For this review, take the finished solid that the model builds, in its own axes (mm). A direction names the side the tool comes from. Round coordinates to 2 decimals unless told otherwise and drop trailing zeros. Loops run counter-clockwise (first coordinate to the right, second up) from the corner with the lowest first, then second, coordinate; pieces in that order, holes last. Notation, with made-up numbers: M 48.25,76.25 L 81.25,76.25 A7 cw 81.25,87.25 Z; hole C 10,85 d7. An arc over 180 degrees is marked long. Write item = value, one per line. Start each with the question number.
```python
from build123d import *

# Parameters (mm, degrees)
BOSS_EXTRUDE1_DEPTH      = 8
BOSS_EXTRUDE1_DEPTH_BACK = 75
SKETCH3_W                = 2.5
SKETCH3_H                = 24
CUT_EXTRUDE1_DEPTH       = 10
BOSS_EXTRUDE6_DEPTH      = 90
BOSS_EXTRUDE6_DEPTH_BACK = 83
BOSS_EXTRUDE7_DEPTH      = 90
SKETCH8_W                = 7
SKETCH8_H                = 16.2
CUT_EXTRUDE2_DEPTH       = 15
SKETCH9_W                = 2
SKETCH9_H                = 12.2
CUT_EXTRUDE3_DEPTH       = 10
CUT_EXTRUDE4_DEPTH       = 90
CUT_EXTRUDE5_DEPTH       = 75
CUT_EXTRUDE6_DEPTH       = 90
CUT_EXTRUDE6_DEPTH_BACK  = 83
SKETCH13_R               = 1.75
SKETCH14_R               = 2
CUT_EXTRUDE7_DEPTH       = 83
SKETCH16_R               = 1.75
CUT_EXTRUDE8_DEPTH       = 3
CUT_EXTRUDE9_DEPTH       = 170
SKETCH18_R               = 2
CUT_EXTRUDE10_DEPTH      = 15
SKETCH19_W               = 8
SKETCH19_H               = 3
CUT_EXTRUDE11_DEPTH      = 3
CUT_EXTRUDE12_DEPTH      = 7
SKETCH21_W               = 7
SKETCH21_H               = 4.5
CUT_EXTRUDE13_DEPTH      = 17
SKETCH22_W               = 40
SKETCH22_H               = 42
CUT_EXTRUDE14_DEPTH      = 42
FILLET1_R                = 5


with BuildPart() as part:
    # Sketch2 → Boss-Extrude1 (new, two sides: drawn at the far end of the back side and taken through both)
    with BuildSketch(Plane(origin=(0, 0, 0), x_dir=(0, 0, -1), z_dir=(1, 0, 0)).offset(-BOSS_EXTRUDE1_DEPTH_BACK)):
        Polygon((-21, 0), (-21, 15), (-4, 15), (-4, 7), (0, 7), (4, 7), (4, 15), (21, 15), (21, 0), (0, 0), align=None)
    extrude(amount=BOSS_EXTRUDE1_DEPTH + BOSS_EXTRUDE1_DEPTH_BACK)

    # Sketch3 → Cut-Extrude1 (cut)
    with BuildSketch(Plane(origin=(0, 15, 0), x_dir=(-1, 0, 0), z_dir=(0, 1, 0))):
        with Locations((-3.75, 0)):
            Rectangle(SKETCH3_W, SKETCH3_H)
    extrude(amount=-CUT_EXTRUDE1_DEPTH, mode=Mode.SUBTRACT)

    # Sketch6 → Boss-Extrude6 (add, two sides: drawn at the far end of the back side and taken through both)
    with BuildSketch(Plane(origin=(8, 0, 0), x_dir=(0, 0, -1), z_dir=(1, 0, 0)).offset(-BOSS_EXTRUDE6_DEPTH_BACK)):
        Polygon((-12, 15), (-12, 0), (12, 0), (12, 15), (21, 15), (21, -27), (-21, -27), (-21, 15), align=None)
    extrude(amount=BOSS_EXTRUDE6_DEPTH + BOSS_EXTRUDE6_DEPTH_BACK)

    # Sketch7 → Boss-Extrude7 (add)
    with BuildSketch(Plane(origin=(8, 0, 0), x_dir=(0, 0, -1), z_dir=(1, 0, 0))):
        Polygon((2.25, 15), (2.25, 8.75), (-2.25, 8.75), (-2.25, 15), (-8.1, 15), (-8.1, 11), (-8.1, 0), (8.1, 0), (8.1, 11), (8.1, 15), align=None)
    extrude(amount=BOSS_EXTRUDE7_DEPTH)

    # Sketch8 → Cut-Extrude2 (cut)
    with BuildSketch(Plane(origin=(0, 15, 0), x_dir=(-1, 0, 0), z_dir=(0, 1, 0))):
        with Locations((-11.5, 0)):
            Rectangle(SKETCH8_W, SKETCH8_H)
    extrude(amount=-CUT_EXTRUDE2_DEPTH, mode=Mode.SUBTRACT)

    # Sketch9 → Cut-Extrude3 (cut)
    with BuildSketch(Plane(origin=(0, 15, 0), x_dir=(-1, 0, 0), z_dir=(0, 1, 0))):
        with Locations((-18, 0)):
            Rectangle(SKETCH9_W, SKETCH9_H)
    extrude(amount=-CUT_EXTRUDE3_DEPTH, mode=Mode.SUBTRACT)

    # Sketch11 → Cut-Extrude4 (cut)
    with BuildSketch(Plane(origin=(98, 0, 0), x_dir=(0, 0, -1), z_dir=(1, 0, 0))):
        with BuildLine():
            Line((4.5, 0), (8.1, 0))
            Line((8.1, 0), (8.1, 0.5))
            Line((8.1, 0.5), (4, 0.5))
            Line((4, 0.5), (4, 0))
            ThreePointArc((4, 0), (0, -4), (-4, 0))
            Line((-4, 0), (-4, 0.5))
            Line((-4, 0.5), (-8.1, 0.5))
            Line((-8.1, 0.5), (-8.1, 0))
            Line((-8.1, 0), (-4.5, 0))
            ThreePointArc((-4.5, 0), (0, -4.5), (4.5, 0))
        make_face()
    extrude(amount=-CUT_EXTRUDE4_DEPTH, mode=Mode.SUBTRACT)

    # Sketch12 → Cut-Extrude5 (cut)
    with BuildSketch(Plane(origin=(98, 0, 0), x_dir=(0, 0, -1), z_dir=(1, 0, 0))):
        with BuildLine():
            Line((-2.25, 15), (-8.1, 15))
            Line((-8.1, 15), (-8.1, 0.5))
            Line((-8.1, 0.5), (-4, 0.5))
            Line((-4, 0.5), (-4, 0))
            ThreePointArc((-4, 0), (0, -4), (4, 0))
            Line((4, 0), (4, 0.5))
            Line((4, 0.5), (8.1, 0.5))
            Line((8.1, 0.5), (8.1, 15))
            Line((8.1, 15), (2.25, 15))
            Line((2.25, 15), (2.25, 8.75))
            Line((2.25, 8.75), (-2.25, 8.75))
            Line((-2.25, 8.75), (-2.25, 15))
        make_face()
    extrude(amount=-CUT_EXTRUDE5_DEPTH, mode=Mode.SUBTRACT)

    # Sketch13 → Cut-Extrude6 (cut, two sides: drawn at the far end of the back side and taken through both)
    with BuildSketch(Plane(origin=(8, 0, 0), x_dir=(0, 0, -1), z_dir=(1, 0, 0)).offset(-CUT_EXTRUDE6_DEPTH_BACK)):
        Circle(SKETCH13_R)
    extrude(amount=CUT_EXTRUDE6_DEPTH + CUT_EXTRUDE6_DEPTH_BACK, mode=Mode.SUBTRACT)

    # Sketch14 → Cut-Extrude7 (cut)
    with BuildSketch(Plane(origin=(8, 0, 0), x_dir=(0, 0, -1), z_dir=(1, 0, 0))):
        Circle(SKETCH14_R)
    extrude(amount=-CUT_EXTRUDE7_DEPTH, mode=Mode.SUBTRACT)

    # Sketch16 → Cut-Extrude8 (cut)
    with BuildSketch(Plane(origin=(98, 0, 0), x_dir=(0, 0, -1), z_dir=(1, 0, 0))):
        with Locations((17.5, -8)):
            Circle(SKETCH16_R)
        with Locations((-17.5, -8)):
            Circle(SKETCH16_R)
    extrude(amount=-CUT_EXTRUDE8_DEPTH, mode=Mode.SUBTRACT)

    # Sketch17 → Cut-Extrude9 (cut)
    with BuildSketch(Plane(origin=(95, 0, 0), x_dir=(0, 0, -1), z_dir=(1, 0, 0))):
        Polygon((18, -6), (18, -27), (-18, -27), (-18, -6), (-4.5, -6), (-4.5, -9), (4.5, -9), (4.5, -6), align=None)
    extrude(amount=-CUT_EXTRUDE9_DEPTH, mode=Mode.SUBTRACT)

    # Sketch18 → Cut-Extrude10 (cut)
    with BuildSketch(Plane(origin=(95, 0, 0), x_dir=(0, 0, -1), z_dir=(1, 0, 0))):
        with Locations((-17.5, -8)):
            Circle(SKETCH18_R)
        with Locations((17.5, -8)):
            Circle(SKETCH18_R)
    extrude(amount=-CUT_EXTRUDE10_DEPTH, mode=Mode.SUBTRACT)

    # Sketch19 → Cut-Extrude11 (cut)
    with BuildSketch(Plane(origin=(95, 0, 0), x_dir=(0, 0, -1), z_dir=(1, 0, 0))):
        with Locations((0, -25.5)):
            Rectangle(SKETCH19_W, SKETCH19_H)
    extrude(amount=CUT_EXTRUDE11_DEPTH, mode=Mode.SUBTRACT)

    # Sketch20 → Cut-Extrude12 (cut)
    with BuildSketch(Plane(origin=(8, 0, 0), x_dir=(0, 0, -1), z_dir=(1, 0, 0))):
        with BuildLine():
            Line((-3.878333303, -1), (3.878323052, -1.000039756))
            ThreePointArc((3.878323052, -1.000039756), (-2.0528e-05, -4.005180297), (-3.878333303, -1))
        make_face()
    extrude(amount=CUT_EXTRUDE12_DEPTH, mode=Mode.SUBTRACT)

    # Sketch21 → Cut-Extrude13 (cut)
    with BuildSketch(Plane(origin=(0, 15, 0), x_dir=(-1, 0, 0), z_dir=(0, 1, 0))):
        with Locations((-11.5, 0)):
            Rectangle(SKETCH21_W, SKETCH21_H)
    extrude(amount=-CUT_EXTRUDE13_DEPTH, mode=Mode.SUBTRACT)

    # Sketch22 → Cut-Extrude14 (cut)
    with BuildSketch(Plane(origin=(0, 15, 0), x_dir=(-1, 0, 0), z_dir=(0, 1, 0))):
        with Locations((55, 0)):
            Rectangle(SKETCH22_W, SKETCH22_H)
    extrude(amount=-CUT_EXTRUDE14_DEPTH, mode=Mode.SUBTRACT)

    # Fillet1
    fillet1_edges = [part.edges().sort_by_distance(p)[0] for p in [
        (31.5, 15, -21),
        (31.5, 15, 21),
        (-35, 15, 12.5),
        (-35, 15, -12.5),
    ]]
    fillet(fillet1_edges, radius=FILLET1_R)


solid = part.part
```
(1) Add section A-A on z = 0. Write out the cut boundary in (x, y), and give its area (3 significant figures).
(2) Draft analysis for pull direction Y (two halves, no side actions). For faces 1 (the flat face through (19, 8, -8.1)), 2 (the flat face through (19, 15, 13)), 3 (the cylindrical face through (96.52, -9.06, -16.11)), 4 (the flat face through (31, -6, -11)), state which applies: +Y half, -Y half, draft (parallel to the pull), parting line (faces both ways), or undercut.
(3) For pin 1 Ø5 at (y, z) = (10, -3.5) entering from +X; pin 2 Ø1 at (x, z) = (16, -1) entering from +Y; pin 3 Ø10 at (x, z) = (-21.5, -11.5) entering from -Y, all flat-tipped, find the tip position at first contact; note any pin that passes through.
(4) Tool access review of faces 5 (the flat face through (96, -26, 4)), 6 (the flat face through (2.5, 6.7, -0.2)), 7 (the flat face through (31, -6, 11)), 8 (the flat face through (6, 11, -4)), 9 (the flat face through (21, 12, -2.25)): name each direction out of +Z, -Z, +X, -X, +Y, -Y from which nothing blocks a thin tool from reaching the whole face with its end or side.
(5) Add section D-D on x = 84. Write out the cut boundary in (y, z), and give its area (3 significant figures).
(6) Add section C-C on y = -14.5. Write out the cut boundary in (x, z), and give its area (3 significant figures).
(7) Add section B-B on x = 11.5. Write out the cut boundary in (y, z), and give its area (3 significant figures).
(8) Wall thickness on L1, parallel to Y at x = 18, z = 0; L2, parallel to X at y = 7, z = 7; L3, parallel to Y at x = 22.5, z = 0: over which ranges is each line inside the solid? List them lowest first.
Answer sheet:
q1.outline = M -35,-9 L 95,-9 L 95,-24 L 98,-24 L 98,-4.5 L 8,-4.5 L 8,-2 L -35,-2 Z; M -35,2 L 8,2 L 8,7 L 5,7 L 5,5 L 2.5,5 L 2.5,7 L -35,7 Z; M 15,-4 L 23,-4 L 23,-1.75 L 15,-1.75 Z; M 15,1.75 L 23,1.75 L 23,8.75 L 19,8.75 L 19,5 L 17,5 L 17,8.75 L 15,8.75 Z
q1.area = 1,030 mm²
q2.face_1 = draft
q2.face_2 = +Y half
q2.face_3 = undercut
q2.face_4 = -Y half
q3.pin_1 = 23
q3.pin_2 = 8.75
q3.pin_3 = -6
q4.face_5 = +X, -X, -Y
q4.face_6 = +Y
q4.face_7 = -X, -Y
q4.face_8 = -X, +Y
q4.face_9 = +X, -X, +Y
q5.outline = M -27,-21 L 10,-21 A5 ccw 15,-16 L 15,-12 L 0,-12 L 0,-4.5 A4.5 cw 0,4.5 L 0,12 L 15,12 L 15,16 A5 ccw 10,21 L -27,21 L -27,18 L -9.94,18 A2 cw -6.06,18 L -6,18 L -6,4.5 L -9,4.5 L -9,-4.5 L -6,-4.5 L -6,-18 L -6.06,-18 A2 cw -9.94,-18 L -27,-18 Z
q5.area = 624 mm²
q6.outline = M -35,-21 L 98,-21 L 98,21 L -35,21 L -35,18 L 95,18 L 95,-18 L -35,-18 Z
q6.area = 906 mm²
q7.outline = M -27,-21 L 10,-21 A5 ccw 15,-16 L 15,-12 L 0,-12 L 0,-4.5 A4.5 cw 0,4.5 L 0,12 L 15,12 L 15,16 A5 ccw 10,21 L -27,21 L -27,18 L -6,18 L -6,4.5 L -9,4.5 L -9,-4.5 L -6,-4.5 L -6,-18 L -27,-18 Z; M -1,-3.87 A4 ccw 0,-4 L 0,-2.25 L -1,-2.25 Z; M -1,2.25 L 0,2.25 L 0,4 A4 ccw -1,3.87 Z
q7.area = 636 mm²
q8.L1 = -9 to -4.5, -4 to -1.75, 1.75 to 5
q8.L2 = -35 to 2.5, 5 to 8, 15 to 23
q8.L3 = -9 to -4.5, -4 to -1.75, 1.75 to 8.75
